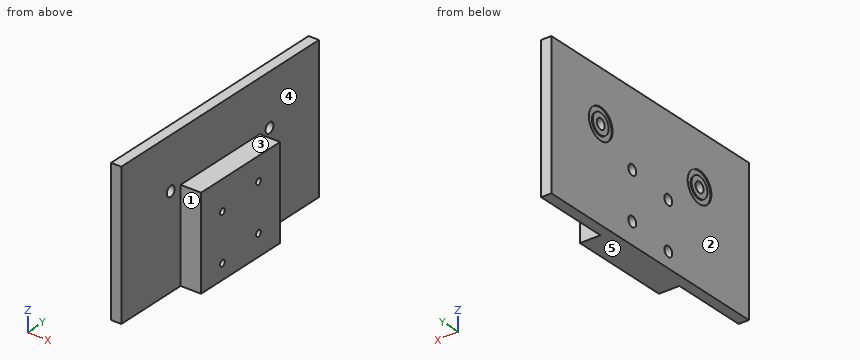
Solid Edge part; units mm, degrees
sketch "Sketch1" plane through (0, 0, 0) normal (0, -1, 0) x (1, 0, 0)
  line L0 (-92.8835, -94.8099) -> (-82.8835, -94.8099)
  line L1 (-82.8835, -94.8099) -> (-82.8835, 45.1901)
  line L2 (-82.8835, 45.1901) -> (-92.8835, 45.1901)
  line L3 (-92.8835, 45.1901) -> (-92.8835, -94.8099)
  dimension "D1" = 82.8835
  dimension "D2" = 92.8835
extrude "Protrusion1" add sketch "Sketch1" against normal blind 250
sketch "Sketch2" plane through (-82.8835, 104, 0.1901) normal (1, 0, 0) x (0, -1, 0)
  line L0 (-71, 5) -> (29, 5)
  line L1 (29, 5) -> (29, 95)
  line L2 (29, 95) -> (-71, 95)
  line L3 (-71, 95) -> (-71, 5)
  dimension "D1" = 71
  dimension "D2" = 71
extrude "Protrusion2" add sketch "Sketch2" along normal blind 20
sketch "Sketch3" plane through (-82.8835, 100, 10.1901) normal (1, 0, 0) x (0, -1, 0)
  circle A0 centre (37.5, 15) radius 5
  circle A1 centre (-87.5, 15) radius 5
extrude "Cutout1" cut sketch "Sketch3" against normal through all
extrude "ExtrudedCutout_6" [suppressed]
sketch "Sketch4" plane through (-92.8835, 145.5, -4.8099) normal (-1, 0, 0) x (0, 1, 0)
  circle A0 centre (2.0953, 68.9118) radius 3
  circle A1 centre (2.0953, 22.9118) radius 3
  circle A2 centre (-43.5, 29) radius 3
  circle A3 centre (-43.5, 75) radius 3
extrude "Cutout2" cut sketch "Sketch4" against normal through all
sketch "Sketch5" plane through (-92.8835, 145.5, 0.1901) normal (-1, 0, 0) x (0, -1, 0)
  circle A0 centre (-2.0953, -73.9118) radius 5
  circle A1 centre (43.5, -80) radius 5
  circle A2 centre (43.5, -34) radius 5
  circle A3 centre (-2.0953, -27.9118) radius 5
extrude "Cutout3" cut sketch "Sketch5" against normal up to vertex (10 mm away)
sketch "Sketch6" plane through (-92.8835, 104, -4.8099) normal (-1, 0, 0) x (0, -1, 0)
  circle A0 centre (41.5, 0) radius 15
  circle A1 centre (-83.5, 0) radius 10
  circle A2 centre (41.5, 0) radius 10
  circle A3 centre (-83.5, 0) radius 15
extrude "ExtrudedCutout_9" cut sketch "Sketch6" against normal blind 1
properties material "Aluminum, 6061-T6"
CAD build for the part. Positions are in the model's coordinates, mm. Face numbers are marked on the shaded views. A direction names the side the tool comes from. Give positions to 0.01 mm unless a question says otherwise; leave off trailing zeros. Loops run counter-clockwise (first coordinate to the right, second up) from the corner with the lowest first, then second, coordinate; pieces in that order, holes last. Notation, with made-up numbers: (-18, -13) -> (2, -13) arc R22 cw to (2, 25) -> close; hole circle Ø8 at (51.25, -20). An arc over 180 degrees is marked (long way). Use a Markdown table: item, result.
1. Slice it at B-B (y = 102). List the corners of the cut face in (x, z), plus the area to 3 significant figures.
Check result:
| item | result |
|---|---|
| outline | (-92.88, -94.81) -> (-62.88, -94.81) -> (-62.88, -82.81) -> (-82.88, -82.81) -> (-82.88, -84.81) -> (-92.88, -84.81) -> close; (-92.88, -74.81) -> (-82.88, -74.81) -> (-82.88, -76.81) -> (-62.88, -76.81) -> (-62.88, -36.81) -> (-82.88, -36.81) -> (-82.88, -38.81) -> (-92.88, -38.81) -> close; (-92.88, -28.81) -> (-82.88, -28.81) -> (-82.88, -30.81) -> (-62.88, -30.81) -> (-62.88, -4.81) -> (-82.88, -4.81) -> (-82.88, 45.19) -> (-92.88, 45.19) -> close |
| area | 2,760 mm^2 |
2. Slice it at D-D (x = -76.5). List the corners of the cut face in (y, z).
Check result:
| item | result |
|---|---|
| outline | (75, -94.81) -> (175, -94.81) -> (175, -4.81) -> (75, -4.81) -> close; hole circle Ø6 at (102, -79.81); hole circle Ø6 at (102, -33.81); hole circle Ø6 at (147.6, -73.72); hole circle Ø6 at (147.6, -27.72) |
3. Flat gauge pins, fed straight in: pin 1 (5 mm diameter, centred on y = 148, z = -28.5, fed in from -X); pin 2 (8 mm diameter, centred on y = 187.5, z = -4.81, fed in from +X); pin 3 (6 mm diameter, centred on x = -68.5, y = 98, fed in from +Z). Where does each tip first touch, or does it go through?
Check result:
| item | result |
|---|---|
| pin 1 | stops at x = -82.88 |
| pin 2 | passes through |
| pin 3 | stops at z = -4.81 |
4. Which spindle directions (+Z, -Z, +X, -X, +Y, -Y) get a long thin tool onto all of the face, cutting with end or side? Do the marked faces 1, 2, 3, 4 and 5. Say none if no direction does.
Check result:
| item | result |
|---|---|
| face 1 | +Z, -Z, +X, -Y |
| face 2 | +Z, -Z, -X, +Y, -Y |
| face 3 | +Z, +X, +Y, -Y |
| face 4 | +Z, +X |
| face 5 | -Z, +X, -X, +Y, -Y |
5. Slice it at C-C (z = -50.5). List the corners of the cut face in (x, y), plus the area to 3 significant figures.
Check result:
| item | result |
|---|---|
| outline | (-92.88, 0) -> (-82.88, 0) -> (-82.88, 75) -> (-62.88, 75) -> (-62.88, 175) -> (-82.88, 175) -> (-82.88, 250) -> (-92.88, 250) -> close |
| area | 4,500 mm^2 |
6. Wall check: L1, parallel to Z at x = -77, y = 102; L2, parallel to Z at x = -92.25, y = 62.5; L3, parallel to Z at x = -74.5, y = 148. Give the ranges that are in metal, low to high. Write a range as [from, to].
Check result:
| item | result |
|---|---|
| L1 | z = [-94.81, -82.81], [-76.81, -36.81], [-30.81, -4.81] |
| L2 | z = [-94.81, -19.81], [-14.81, -9.81], [0.19, 5.19], [10.19, 45.19] |
| L3 | z = [-94.81, -76.69], [-70.75, -30.69], [-24.75, -4.81] |
7. Slice it at A-A (y = 187.5). List the corners of the cut face in (x, z).
Check result:
| item | result |
|---|---|
| outline | (-92.88, -94.81) -> (-82.88, -94.81) -> (-82.88, -9.81) -> (-92.88, -9.81) -> (-92.88, -14.81) -> (-91.88, -14.81) -> (-91.88, -19.81) -> (-92.88, -19.81) -> close; (-92.88, 0.19) -> (-82.88, 0.19) -> (-82.88, 45.19) -> (-92.88, 45.19) -> (-92.88, 10.19) -> (-91.88, 10.19) -> (-91.88, 5.19) -> (-92.88, 5.19) -> close |
